The listing builds one solid part. Answer for the finished solid, in the listing's coordinates (mm). A direction names the side the tool comes from. Round coordinates to 2 decimals unless told otherwise and drop trailing zeros. Write each loop counter-clockwise with the first axis right and the second up, starting at its lowest first coordinate (ties: lowest second). Pieces come first, ordered by that corner, then holes. Notation, with made-up numbers: (26, 73) - (39, 73) arc R11 cw to (39, 79) - close; hole circle Ø3 at (15, 7.5). An arc over 180 degrees is marked (long way). Return JSON: item names as keys, results as strings. Group by question number.
Autodesk Fusion 360 part; units mm, degrees
sketch "Sketch1" plane through (0, 0, 0) normal (0, 0, 1) x (1, 0, 0)
  line L0 (61.321, 25.4) -> (25.4, 61.321)
  line L1 (25.4, 61.321) -> (-25.4, 61.321)
  line L2 (-25.4, 61.321) -> (-61.321, 25.4)
  line L3 (-61.321, 25.4) -> (-61.321, -25.4)
  line L4 (-61.321, -25.4) -> (-25.4, -61.321)
  line L5 (-25.4, -61.321) -> (25.4, -61.321)
  line L6 (25.4, -61.321) -> (61.321, -25.4)
  line L7 (61.321, -25.4) -> (61.321, 25.4)
  dimension "d1" = 50.8
extrude "Extrude1" add sketch "Sketch1" along normal blind 38.1
sketch "Sketch6" plane through (0, 0, 38.1) normal (0, 0, 1) x (-1, 0, 0)
  line L0 (-61.321, 25.4) -> (-61.321, -25.4)
  line L1 (-61.321, -25.4) -> (-25.4, -61.321)
  line L2 (-25.4, -61.321) -> (25.4, -61.321)
  line L3 (25.4, -61.321) -> (61.321, -25.4)
  line L4 (61.321, -25.4) -> (61.321, 25.4)
  line L5 (61.321, 25.4) -> (25.4, 61.321)
  line L6 (25.4, 61.321) -> (-25.4, 61.321)
  line L7 (-25.4, 61.321) -> (-61.321, 25.4)
  line L8 (-12.8905, 9.017) -> (12.8905, 9.017)
  line L9 (12.8905, 9.017) -> (12.8905, -9.017)
  line L10 (12.8905, -9.017) -> (-12.8905, -9.017)
  line L11 (-12.8905, -9.017) -> (-12.8905, 9.017)
  line L12 (-12.8905, 9.017) -> (12.8905, -9.017) construction
  line L13 (12.8905, 9.017) -> (-12.8905, -9.017) construction
  dimension "d28" = 25.781
  dimension "d29" = 18.034
extrude "Extrude12" cut sketch "Sketch6" against normal blind 19.05 contours L8 L9 L10 L11
sketch "Sketch7" plane through (0, 0, 19.05) normal (0, 0, 1) x (-1, 0, 0)
  line L0 (-12.8905, -9.017) -> (12.8905, -9.017)
  line L1 (12.8905, -9.017) -> (12.8905, 9.017)
  line L2 (12.8905, 9.017) -> (-12.8905, 9.017)
  line L3 (-12.8905, 9.017) -> (-12.8905, -9.017)
  circle A0 centre (10.16, -6.35) radius 0.85
  dimension "d40" = 1.7
  dimension "d41" = 10.16
  dimension "d42" = 6.35
extrude "Extrude13" cut sketch "Sketch7" against normal blind 6.35 contours A0
sketch "Sketch8" plane through (0, 0, 19.05) normal (0, 0, 1) x (-1, 0, 0)
  circle A0 centre (10.16, -6.35) radius 0.85
  line L0 (-12.8905, -9.017) -> (12.8905, -9.017)
  line L1 (12.8905, -9.017) -> (12.8905, 9.017)
  line L2 (12.8905, 9.017) -> (-12.8905, 9.017)
  line L3 (-12.8905, 9.017) -> (-12.8905, -9.017)
  line L4 (0, -11.43) -> (0, 10.8522)
  line L5 (13.97, 0) -> (-13.97, 0)
  circle A1 centre (-10.16, -6.35) radius 0.85
  circle A2 centre (10.16, 6.35) radius 0.85
  circle A3 centre (-10.16, 6.35) radius 0.85
extrude "Extrude14" cut sketch "Sketch8" against normal blind 6.35 contours A1 | A2 | A3
sketch "Sketch9" plane through (0, 0, 19.05) normal (0, 0, 1) x (-1, 0, 0)
  circle A0 centre (-10.16, -6.35) radius 0.85
  circle A1 centre (-10.16, 6.35) radius 0.85
  circle A2 centre (10.16, 6.35) radius 0.85
  circle A3 centre (10.16, -6.35) radius 0.85
  line L0 (-12.8905, -9.017) -> (12.8905, -9.017)
  line L1 (12.8905, -9.017) -> (12.8905, 9.017)
  line L2 (12.8905, 9.017) -> (-12.8905, 9.017)
  line L3 (-12.8905, 9.017) -> (-12.8905, -9.017)
  line L4 (7.874, 5.0932) -> (-7.874, 5.0932)
  line L5 (-7.874, 5.0932) -> (-7.874, 8.2682)
  line L6 (-7.874, 8.2682) -> (7.874, 8.2682)
  line L7 (7.874, 8.2682) -> (7.874, 5.0932)
  dimension "d45" = 15.748
  dimension "d46" = 3.175
  dimension "d47" = 7.874
extrude "Extrude15" cut sketch "Sketch9" against normal blind 5.08 contours L4 L5 L6 L7
sketch "Sketch10" plane through (0, 0, 38.1) normal (0, 0, 1) x (-1, 0, 0)
  line L0 (12.8905, 9.017) -> (12.8905, -9.017)
  line L1 (12.8905, -9.017) -> (-12.8905, -9.017)
  line L2 (-12.8905, -9.017) -> (-12.8905, 9.017)
  line L3 (-12.8905, 9.017) -> (12.8905, 9.017)
  line L4 (-61.321, 25.4) -> (-61.321, -25.4)
  line L5 (-61.321, -25.4) -> (-25.4, -61.321)
  line L6 (-25.4, -61.321) -> (25.4, -61.321)
  line L7 (25.4, -61.321) -> (61.321, -25.4)
  line L8 (61.321, -25.4) -> (61.321, 25.4)
  line L9 (61.321, 25.4) -> (25.4, 61.321)
  line L10 (25.4, 61.321) -> (-25.4, 61.321)
  line L11 (-25.4, 61.321) -> (-61.321, 25.4)
  line L12 (41.275, -36.068) -> (-41.275, -36.068)
  line L13 (-41.275, -36.068) -> (-41.275, -15.24)
  line L14 (-41.275, -15.24) -> (41.275, -15.24)
  line L15 (41.275, -15.24) -> (41.275, -36.068)
  line L16 (41.275, -36.068) -> (-41.275, -15.24) construction
  line L17 (-41.275, -36.068) -> (41.275, -15.24) construction
  point P0 (0, -25.654)
  dimension "d50" = 82.55
  dimension "d51" = 20.828
  dimension "d52" = 15.24
extrude "Extrude16" cut sketch "Sketch10" against normal blind 19.05 contours L12 L13 L14 L15
equation "d47 = ( 0.62 / 2 ) * 1 in"
(1) Find section A-A (z = 11). Write down the section's boundary in (x, y), plus the area to 3 significant figures.
(2) Find section C-C (z = 22.5). Write down the section's boundary in (x, y) (1 decimal).
(3) Consider line 1 (Y direction, x = -10, z = 15); line 2 (X direction, y = 6.35, z = 15.25); line 3 (X direction, y = -6.35, z = 14.25). Determine where each line is inside the solid, lowest interval first.
(4) Determine the mould class of faces 1 (the flat face through (-43.61, -43.11, 18.78)), 2 (the flat face through (1, 15.24, 29)), 3 (the flat face through (0, 61.321, 19)), 4 (the flat face through (41.275, 26, 29)) for opening direction X: +X half, -X half, draft (parallel to the pull), parting line (faces both ways), or undercut.
(5) Flat-ended cylindrical pins translate along their axes: pin 1 (0.8 mm diameter, centred on x = 10, y = 6.5, fed in from +Z); pin 2 (1.5 mm diameter, centred on y = 32, z = 6, fed in from -X); pin 3 (1.9 mm diameter, centred on x = 10.5, y = -6.5, fed in from +Z). Find the tip coordinate at first contact, or state that the pin passes through.
(6) Find section B-B (y = 23). Write down the section's boundary in (x, z) (3 decimals), plus the area to 3 significant figures.
(7) For faces 5 (the flat face through (43.61, 43.11, 18.78)), 6 (the flat face through (-12.89, 0, 29)), determine the directions among +Z, -Z, +X, -X, +Y, -Y from which every point of the face is accessible in a straight line to the end or side of a thin tool.
(8) Find section D-D (x = 4). Write down the section's boundary in (y, z), plus the area to 3 significant figures.
Check sheet entries:
{
 "1": {"outline": "(-61.32, -25.4) - (-25.4, -61.32) - (25.4, -61.32) - (61.32, -25.4) - (61.32, 25.4) - (25.4, 61.32) - (-25.4, 61.32) - (-61.32, 25.4) - close", "area": "12,500 mm^2"},
 "2": {"outline": "(-61.3, -25.4) - (-25.4, -61.3) - (25.4, -61.3) - (61.3, -25.4) - (61.3, 25.4) - (25.4, 61.3) - (-25.4, 61.3) - (-61.3, 25.4) - close; hole (-41.3, 15.2) - (41.3, 15.2) - (41.3, 36.1) - (-41.3, 36.1) - close; hole (-12.9, -9) - (12.9, -9) - (12.9, 9) - (-12.9, 9) - close"},
 "3": {"line 1": "y = -61.32 to -7.18, -5.52 to 5.52, 7.18 to 61.32", "line 2": "x = -61.32 to -11.01, -9.31 to 9.31, 11.01 to 61.32", "line 3": "x = -61.32 to -11.01, -9.31 to -7.87, 7.87 to 9.31, 11.01 to 61.32"},
 "4": {"face 1": "-X half", "face 2": "undercut", "face 3": "draft", "face 4": "undercut"},
 "5": {"pin 1": "stops at z = 12.7", "pin 2": "stops at x = -55.47", "pin 3": "stops at z = 19.05"},
 "6": {"outline": "(-61.321, 0) - (61.321, 0) - (61.321, 38.1) - (41.275, 38.1) - (41.275, 19.05) - (-41.275, 19.05) - (-41.275, 38.1) - (-61.321, 38.1) - close", "area": "3,100 mm^2"},
 "7": {"face 5": "+Z, -Z, +X, +Y", "face 6": "+Z"},
 "8": {"outline": "(-61.32, 0) - (61.32, 0) - (61.32, 38.1) - (36.07, 38.1) - (36.07, 19.05) - (15.24, 19.05) - (15.24, 38.1) - (9.02, 38.1) - (9.02, 19.05) - (-5.09, 19.05) - (-5.09, 13.97) - (-8.27, 13.97) - (-8.27, 19.05) - (-9.02, 19.05) - (-9.02, 38.1) - (-61.32, 38.1) - close", "area": "3,920 mm^2"}
}
